Geometry: final body of the model. Coordinates: model frame, mm. Round coordinates to 2 decimals unless told otherwise and drop trailing zeros. Loops run counter-clockwise (first coordinate to the right, second up) from the corner with the lowest first, then second, coordinate; pieces in that order, holes last. Notation, with made-up numbers: M -37.75,-32.75 L 8.25,-32.75 A18 ccw 8.25,-10.75 Z; hole C 32,54.5 d1. An arc over 180 degrees is marked long. Answer as a JSON object with one key per item and string values.
from build123d import *

# Parameters (mm, degrees)
F1_DEPTH  = 6.35
F3_DEPTH  = 0.254
F4_R      = 1.27
F5_W      = 66.04
F5_H      = 114.3
F6_DEPTH  = 0.0254
F8_W      = 1.5875
F8_H      = 22.225
F9_DEPTH  = 0.0254
F11_R     = 1.524
F12_DEPTH = 25.4


with BuildPart() as f1:
    # F0 (on Front) → F1 (new body)
    with BuildSketch(Plane.XZ):
        with BuildLine():
            Line((59.69, 0), (12.7, 0))
            ThreePointArc((12.7, 0), (3.7197438789, -3.7197438789), (0, -12.7))
            Line((0, -12.7), (0, -127))
            ThreePointArc((0, -127), (3.7197438789, -135.9802561211), (12.7, -139.7))
            Line((12.7, -139.7), (59.69, -139.7))
            ThreePointArc((59.69, -139.7), (68.6702561211, -135.9802561211), (72.39, -127))
            Line((72.39, -127), (72.39, -12.7))
            ThreePointArc((72.39, -12.7), (68.6702561211, -3.7197438789), (59.69, 0))
        make_face()
    extrude(amount=F1_DEPTH)

    # F2 (on face) → F3 (join)
    with BuildSketch(Plane.XZ.offset(6.35)):
        with BuildLine():
            Line((41.8465, -131.1656), (30.5435, -131.1656))
            ThreePointArc((30.5435, -131.1656), (28.2575, -133.4516), (30.5435, -135.7376))
            Line((30.5435, -135.7376), (41.8465, -135.7376))
            ThreePointArc((41.8465, -135.7376), (44.1325, -133.4516), (41.8465, -131.1656))
        make_face()
    extrude(amount=F3_DEPTH)

    # F4
    f4_edges = [f1.edges().sort_by_distance(p)[0] for p in [
        (72.39, -6.35, -69.85),
        (72.39, 0, -69.85),
    ]]
    fillet(f4_edges, radius=F4_R)

    # F5 (on face) → F6 (cut)
    with BuildSketch(Plane.XZ.offset(6.35)):
        with Locations((36.195, -70.8406)):
            Rectangle(F5_W, F5_H)
    extrude(amount=-F6_DEPTH, mode=Mode.SUBTRACT)

    # F8 (on offset) → F9 (join)
    with BuildSketch(Plane(origin=(0, 0, 0), x_dir=(0, -1, 0), z_dir=(-1, 0, 0))):
        with Locations((3.19405, -30.1625)):
            Rectangle(F8_W, F8_H)
    extrude(amount=F9_DEPTH)

    # F11 (on offset) → F12 (cut)
    with BuildSketch(Plane.XY):
        with Locations((61.3411824728, -3.2385)):
            Circle(F11_R)
    extrude(amount=-F12_DEPTH, mode=Mode.SUBTRACT)


solid = f1.part
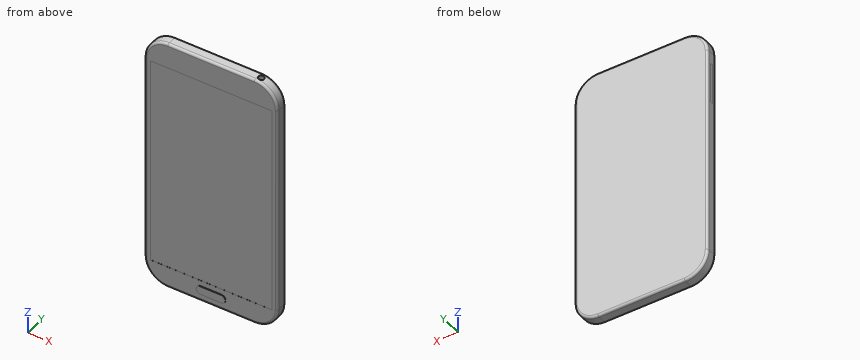
1) Pin query (flat end, axial travel): P1, Ø1, axis at x = 7.5, z = -23, coming from the -Y side; P2, Ø1.9, axis at y = -3, z = -84.5, coming from the -X side. Return the tip coordinate at first contact, or that it passes through.
Results:
{"P1": "y = -6.32", "P2": "x = 0"}
2) Section query A-A (z = -60). Return the cut outline in (x, y) (3 decimals), and give its area (3 significant figures).
Results:
{"outline": "M 0,-5.08 A1.27 ccw 1.27,-6.35 L 3.175,-6.35 L 3.175,-6.325 L 69.215,-6.325 L 69.215,-6.35 L 71.12,-6.35 A1.27 ccw 72.39,-5.08 L 72.39,-1.27 A1.27 ccw 71.12,0 L 1.27,0 A1.27 ccw 0,-1.27 Z", "area": "457 mm2"}
3) Ray query, line 1 (Y direction, x = 15.5, z = -65.5); line 2 (X direction, y = -1.25, z = -32.5); line 3 (Y direction, x = 37, z = -12.5). Return the intervals inside material, ascending.
Results:
{"line 1": "-6.32 to 0", "line 2": "0 to 72.39", "line 3": "-6.35 to 0"}
